Geometry: see drawing. Coordinates: mm, zero at the bounding-box minimum. Coordinates: 2 decimals unless noted, no trailing zeros. Loops run counter-clockwise (first coordinate to the right, second up) from the corner with the lowest first, then second, coordinate; pieces in that order, holes last. Notation, with made-up numbers: (-4.75, 0.5) -> (49.25, 0.5) arc R28 ccw to (49.25, 35.5) -> close; hole circle Ø6 at (78.5, 6). An arc over 180 degrees is marked (long way). One line per question, with ' | ' between items. Start each with the question number.
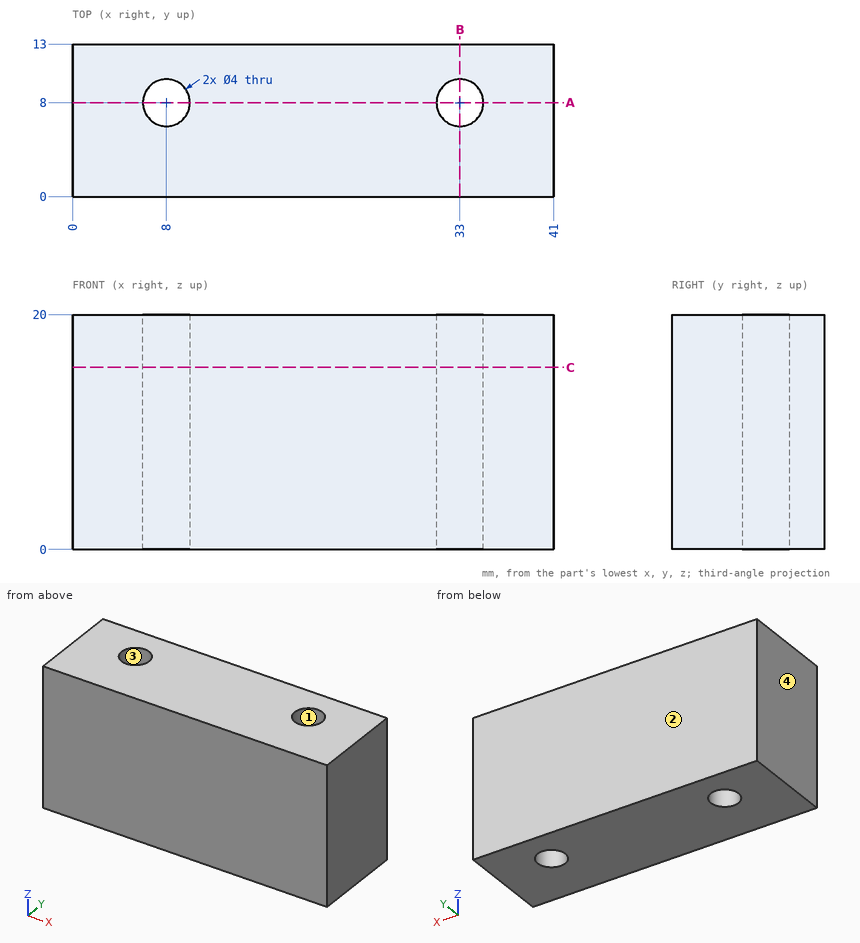
(1) Cut plane A-A, the plane y = 8. Return the cut outline in (x, z), and give its area (3 significant figures).
(2) Ray query, L1, parallel to X at y = 7.25, z = 18.5; L2, parallel to Y at x = 8, z = 8.5; L3, parallel to Y at x = 32, z = 11.5. Return the intervals inside material, ascending.
(3) Draft query along X for the marked faces 1, 2, 3 and 4. Return one class per face: pulls with the +X half, pulls with the -X half, needs draft (parallel to the pull), parting line crosses it, or undercut.
(4) Cut plane B-B, the plane x = 33. Return the cut outline in (y, z), and give its area (3 significant figures).
(5) Cut plane C-C, the plane z = 15.5. Return the cut outline in (x, y), and give its area (3 significant figures).
Here are the results:
1) outline: (0, 0) -> (6, 0) -> (6, 20) -> (0, 20) -> close; (10, 0) -> (31, 0) -> (31, 20) -> (10, 20) -> close; (35, 0) -> (41, 0) -> (41, 20) -> (35, 20) -> close | area: 660 mm2
2) L1: x = 0 to 6.15, 9.85 to 31.15, 34.85 to 41 | L2: y = 0 to 6, 10 to 13 | L3: y = 0 to 6.27, 9.73 to 13
3) face 1: undercut | face 2: needs draft | face 3: undercut | face 4: pulls with the -X half
4) outline: (0, 0) -> (6, 0) -> (6, 20) -> (0, 20) -> close; (10, 0) -> (13, 0) -> (13, 20) -> (10, 20) -> close | area: 180 mm2
5) outline: (0, 0) -> (41, 0) -> (41, 13) -> (0, 13) -> close; hole circle Ø4 at (8, 8); hole circle Ø4 at (33, 8) | area: 508 mm2
